from build123d import *

# Parameters (mm, degrees)
EXTRUDE1_DEPTH        = 1
SKETCH2_W             = 165
SKETCH2_H             = 32
CUT_EXTRUDE1_DEPTH    = 1
SKETCH3_R             = 6.5
SKETCH3_R_2           = 5.25
CUT_EXTRUDE2_DEPTH    = 1
ESBO_O1_R             = 1.6
CORTE_EXTRUS_O1_DEPTH = 2


with BuildPart() as part:
    # Sketch1 → Extrude1 (new body)
    with BuildSketch(Plane.XY):
        Polygon((-122, 84), (122, 84), (122, 76), (130, 76), (130, 66), (138, 66), (138, -66), (130, -66), (130, -76), (122, -76), (122, -84), (-122, -84), (-122, -76), (-130, -76), (-130, -66), (-138, -66), (-138, 66), (-130, 66), (-130, 76), (-122, 76), align=None)
    extrude(amount=EXTRUDE1_DEPTH)

    # Sketch2 → Cut-Extrude1 (cut)
    with BuildSketch(Plane.XY.offset(1)):
        with Locations((-7.5, 28.75)):
            Rectangle(SKETCH2_W, SKETCH2_H)
    extrude(amount=-CUT_EXTRUDE1_DEPTH, mode=Mode.SUBTRACT)

    # Sketch3 → Cut-Extrude2 (cut)
    with BuildSketch(Plane.XY.offset(1)):
        with Locations((-105.5, 53.5)):
            Circle(SKETCH3_R)
        with Locations((-105.5, 28.75)):
            Circle(SKETCH3_R)
        with Locations((-48.5, 3.5)):
            Circle(SKETCH3_R)
        with Locations((2.5, 3.5)):
            Circle(SKETCH3_R)
        with Locations((53.5, 3.5)):
            Circle(SKETCH3_R)
        with Locations((53.5, 53.5)):
            Circle(SKETCH3_R)
        with Locations((2.5, 53.5)):
            Circle(SKETCH3_R)
        with Locations((-48.5, 53.5)):
            Circle(SKETCH3_R)
        with Locations((96.873262634, 38.092814818)):
            Circle(SKETCH3_R_2)
        with Locations((109.5, 35)):
            Circle(SKETCH3_R_2)
        with Locations((109.5, 22)):
            Circle(SKETCH3_R_2)
        with Locations((96.873262634, 22)):
            Circle(SKETCH3_R_2)
    extrude(amount=-CUT_EXTRUDE2_DEPTH, mode=Mode.SUBTRACT)

    # Esboço1 → Corte-extrusão1 (cut, through all)
    with BuildSketch(Plane.XY.offset(1)):
        with Locations((0, -80.5)):
            Circle(ESBO_O1_R)
        with Locations((-100, -80.5)):
            Circle(ESBO_O1_R)
        with Locations((100, -80.5)):
            Circle(ESBO_O1_R)
        with Locations((-135, 0)):
            Circle(ESBO_O1_R)
        with Locations((135, 0)):
            Circle(ESBO_O1_R)
        with Locations((100, 80.5)):
            Circle(ESBO_O1_R)
        with Locations((-100, 80.5)):
            Circle(ESBO_O1_R)
        with Locations((0, 80.5)):
            Circle(ESBO_O1_R)
    extrude(amount=-CORTE_EXTRUS_O1_DEPTH, mode=Mode.SUBTRACT)


solid = part.part
Geometry check sheet. Reference: the model listing, model coordinates, mm. Give positions to 0.01 mm unless a question says otherwise; leave off trailing zeros. Write each loop counter-clockwise with the first axis right and the second up, starting at its lowest first coordinate (ties: lowest second). Pieces come first, ordered by that corner, then holes. Notation, with made-up numbers: M -12.75,36 L -0.75,36 A11 ccw -0.75,42 Z; hole C 34,62.25 d3. An arc over 180 degrees is marked long. One line per question, with ' | ' between items.
1. Cross-section at B-B (x = 109.5). Enter the section's corners in (y, z).
Ans:
outline: M -84,0 L 16.75,0 L 16.75,1 L -84,1 Z; M 27.25,0 L 29.75,0 L 29.75,1 L 27.25,1 Z; M 40.25,0 L 84,0 L 84,1 L 40.25,1 Z
2. Cross-section at D-D (y = 7). Enter the section's corners in (x, z).
Ans:
outline: M -138,0 L -53.98,0 L -53.98,1 L -138,1 Z; M -43.02,0 L -2.98,0 L -2.98,1 L -43.02,1 Z; M 7.98,0 L 48.02,0 L 48.02,1 L 7.98,1 Z; M 58.98,0 L 138,0 L 138,1 L 58.98,1 Z
3. Cross-section at C-C (x = -48.5). Enter the section's corners in (y, z).
Ans:
outline: M -84,0 L -3,0 L -3,1 L -84,1 Z; M 10,0 L 12.75,0 L 12.75,1 L 10,1 Z; M 44.75,0 L 47,0 L 47,1 L 44.75,1 Z; M 60,0 L 84,0 L 84,1 L 60,1 Z
4. Cross-section at A-A (x = -85.5). Enter the section's corners in (y, z).
Ans:
outline: M -84,0 L 12.75,0 L 12.75,1 L -84,1 Z; M 44.75,0 L 84,0 L 84,1 L 44.75,1 Z
5. Mould release check, pull along X, two halves, no side actions. Record for faces 1 (the face through (2, -17, 1)), 2 (the face through (-2.658, -0.455, 0.507)): released by +X, released by -X, zero draft, split by the parting line, or undercut.
Ans:
face 1: zero draft | face 2: undercut
6. Scan lines: line 1 along Y through (x, z) = (-48.5, 0.6); line 2 along Y through (x, z) = (109.5, 0.9); line 3 along X through (y, z) = (-80.5, 0.6). Record each from-to range of solid material in increasing order. Write a range as from..to.
Ans:
line 1: -84..-3, 10..12.75, 44.75..47, 60..84 | line 2: -84..16.75, 27.25..29.75, 40.25..84 | line 3: -122..-101.6, -98.4..-1.6, 1.6..98.4, 101.6..122
